Autodesk Fusion 360 part; units mm, degrees
ref_plane "WorkPlane1" through (0, 0, 0) normal (0, 0, 1) x (1, 0, 0)
sketch "Sketch1" plane through (0, 0, 0) normal (0, 0, 1) x (1, 0, 0)
  line L0 (10.25, 10.25) -> (-10.25, 10.25)
  line L1 (-10.25, 10.25) -> (-10.25, -10.25)
  line L2 (-10.25, -10.25) -> (10.25, -10.25)
  line L3 (10.25, -10.25) -> (10.25, 10.25)
  line L4 (10.25, 10.25) -> (-10.25, -10.25) construction
  line L5 (-10.25, 10.25) -> (10.25, -10.25) construction
  line L6 (3.75, 3.75) -> (-3.75, 3.75)
  line L7 (-3.75, 3.75) -> (-3.75, -3.75)
  line L8 (-3.75, -3.75) -> (3.75, -3.75)
  line L9 (3.75, -3.75) -> (3.75, 3.75)
  line L10 (3.75, 3.75) -> (-3.75, -3.75) construction
  line L11 (-3.75, 3.75) -> (3.75, -3.75) construction
  line L12 (8.1, 8.1) -> (-8.1, 8.1)
  line L13 (-8.1, 8.1) -> (-8.1, -8.1)
  line L14 (-8.1, -8.1) -> (8.1, -8.1)
  line L15 (8.1, -8.1) -> (8.1, 8.1)
  line L16 (8.1, 8.1) -> (-8.1, -8.1) construction
  line L17 (-8.1, 8.1) -> (8.1, -8.1) construction
  line L18 (10.25, 10.25) -> (5.55, 10.25)
  line L19 (5.55, 10.25) -> (5.55, 5.55)
  line L20 (5.55, 5.55) -> (10.25, 5.55)
  line L21 (10.25, 5.55) -> (10.25, 10.25)
  line L22 (2.7601, 3.75) -> (5.55, 6.5399)
  line L23 (3.75, 2.7601) -> (6.5399, 5.55)
  line L24 (4.155, 5.145) -> (5.145, 4.155)
  line L25 (-5.55, 5.55) -> (-5.55, 10.25)
  line L26 (-10.25, 5.55) -> (-5.55, 5.55)
  line L27 (-3.75, 2.7601) -> (-6.5399, 5.55)
  line L28 (-2.7601, 3.75) -> (-5.55, 6.5399)
  line L29 (-5.55, -5.55) -> (-10.25, -5.55)
  line L30 (-5.55, -10.25) -> (-5.55, -5.55)
  line L31 (-2.7601, -3.75) -> (-5.55, -6.5399)
  line L32 (-3.75, -2.7601) -> (-6.5399, -5.55)
  line L33 (5.55, -5.55) -> (5.55, -10.25)
  line L34 (10.25, -5.55) -> (5.55, -5.55)
  line L35 (3.75, -2.7601) -> (6.5399, -5.55)
  line L36 (2.7601, -3.75) -> (5.55, -6.5399)
  point P0 (4.65, 4.65)
  dimension "d2" = 20.5
  dimension "d3" = 20.5
  dimension "d4" = 7.5
  dimension "d5" = 7.5
  dimension "d6" = 16.2
  dimension "d7" = 16.2
  dimension "d8" = 4.7
  dimension "d9" = 4.7
  dimension "d10" = 1.4
  dimension "d12" = 360
extrude "Extrude1" add sketch "Sketch1" against normal blind 5 makes body 1
extrude "Extrude2" add sketch "Sketch1" along normal blind 10 draft -1 separate body contours L6 L12 L19 L22 L25 L28 makes body 2
sketch "Sketch2" plane through (0, 0, -5) normal (0, 0, -1) x (1, 0, 0)
  line L0 (10.25, -10.25) -> (10.25, 10.25)
  line L1 (10.25, 10.25) -> (-10.25, 10.25)
  line L2 (-10.25, 10.25) -> (-10.25, -10.25)
  line L3 (-10.25, -10.25) -> (10.25, -10.25)
  circle A0 centre (0, 0) radius 2.1
  line L4 (2.0063, 3.475) -> (-2.0063, 3.475)
  line L5 (-2.0063, 3.475) -> (-4.0126, 0)
  line L6 (-4.0126, 0) -> (-2.0063, -3.475)
  line L7 (-2.0063, -3.475) -> (2.0063, -3.475)
  line L8 (2.0063, -3.475) -> (4.0126, 0)
  line L9 (4.0126, 0) -> (2.0063, 3.475)
  dimension "d17" = 4.2
  dimension "d18" = 3.475
extrude "Extrude3" cut sketch "Sketch2" against normal up to surface (5 mm away) contours A0 bodies 2
extrude "Extrude4" cut sketch "Sketch2" against normal blind 3 contours L4 L5 L6 L7 L8 L9 bodies 1
fillet "Fillet1" radius 0.5 6 edges at (2.7239, 3.8373, 5) (-2.7239, 3.8373, 5) (-5.4627, 6.5761, 5) (5.4627, 6.5761, 5) (5.4627, 8.0127, 5) (-5.4627, 8.0127, 5) on bodies 2
pattern_circular "C-Pattern1" count 4 over 360 about axis through (0, 0, 1.75) along (0, 0, 1) of bodies 2 makes body 3 at (-8.0418, 1.6252, 3.3333) makes body 4 at (-1.6252, -8.0418, 3.3333) makes body 5 at (8.0418, -1.6252, 3.3333)
combine "Combine1" operation add target body 5 tool bodies 4 3 2 1
fillet "Fillet2" radius 0.2 4 edges at (10.25, -10.25, -2.5) (10.25, 10.25, -2.5) (-10.25, 10.25, -2.5) (-10.25, -10.25, -2.5) on bodies 5
equation "d18 = ( 6.95 / 2 ) * 1 mm"
Check sheet for the modelled part. Datum: model origin and axes. Units: mm. A direction names the side the tool comes from. Give positions to 0.01 mm unless a question says otherwise; leave off trailing zeros. Write each loop counter-clockwise with the first axis right and the second up, starting at its lowest first coordinate (ties: lowest second). Pieces come first, ordered by that corner, then holes. Notation, with made-up numbers: M 24,43 L 81,43 A21 ccw 81,69 Z; hole C 37.5,-21 d8. An arc over 180 degrees is marked long. Use one line per item in the form item = value.
(1) Material ranges on line 1 along Y through (x, z) = (5, 8.5); line 2 along X through (y, z) = (-4.75, 7.5); line 3 along Z through (x, y) = (8.25, -6), recorded low to high.
Answer block:
line_1 = -7.94 to -6.2, -3.8 to 3.8, 6.2 to 7.94
line_2 = -7.97 to -5.93, -3.57 to 3.57, 5.93 to 7.97
line_3 = -5 to 0
(2) Draft check along X on faces 3 (the flat face through (0, 0, -5)), 4 (the flat face through (2.995, 1.762, -3.521)). Enter one of: pulls with the +X half, pulls with the -X half, needs draft (parallel to the pull), parting line crosses it, or undercut.
Answer block:
face_3 = needs draft
face_4 = undercut
(3) Section check A-A on x = 0. Record the boundary of the cut face in (y, z) (3 decimals), plus the area to 3 significant figures.
Answer block:
outline = M -10.25,-5 L -3.475,-5 L -3.475,-2 L -2.1,-2 L -2.1,-5 L 2.1,-5 L 2.1,-2 L 3.475,-2 L 3.475,-5 L 10.25,-5 L 10.25,0 L 8.1,0 L 7.925,10 L 3.925,10 L 3.75,0 L -3.75,0 L -3.925,10 L -7.925,10 L -8.1,0 L -10.25,0 Z
area = 178 mm2
(4) Tool access check on faces 1 (the flat face through (-5, 0, -5)), 2 (the flat face through (-2.995, -1.762, -3.521)). Record the directions out of +Z, -Z, +X, -X, +Y, -Y that give a thin tool (end or side, any length) a straight path to the whole face; none if there is none.
Answer block:
face_1 = -Z, +X, -X, +Y, -Y
face_2 = -Z
(5) Section check B-B on y = -8.5. Record the boundary of the cut face in (x, z).
Answer block:
outline = M -10.25,-5 L 10.25,-5 L 10.25,0 L -10.25,0 Z
(6) Depth check by flat-ended pin: P1, Ø1.5, axis at y = 1.5, z = 8, coming from the -X side. Enter the tip coordinate at first touch or a pass-through.
Answer block:
P1 = -7.97
(7) Section check C-C on z = 4.75. State how many separate pieces and enclosed holes the cut face has, plus the area to 3 significant figures.
Answer block:
separate_pieces = 4
enclosed_holes = 0
area = 152 mm2
